For this review, take the finished solid that the model builds, in its own axes (mm). A direction names the side the tool comes from. Round coordinates to 2 decimals unless told otherwise and drop trailing zeros. Loops run counter-clockwise (first coordinate to the right, second up) from the corner with the lowest first, then second, coordinate; pieces in that order, holes last. Notation, with made-up numbers: (49, -31) -> (74, -31) arc R10 cw to (74, -27) -> close; hole circle Ø9 at (75.25, -29.75). An arc over 180 degrees is marked (long way). Use one line per item in the form item = value. Start each with the question number.
Autodesk Inventor part; units mm, degrees
sketch "Sketch1" plane through (0, 0, 0) normal (0, 0, 1) x (1, 0, 0)
  line L0 (0, 2.868) -> (2, 2.868)
  line L1 (2, 2.868) -> (2, -21.132)
  line L2 (2, -21.132) -> (0, -21.132)
  line L3 (0, -21.132) -> (0, 2.868)
  line L4 (4, -23.132) -> (4, 4.868)
  line L5 (4, 4.868) -> (0, 4.868)
  line L6 (0, -23.132) -> (4, -23.132)
  line L7 (0, 2.868) -> (0, 4.868)
  line L8 (0, -23.132) -> (0, -21.132)
  line L9 (-30, 5.364) -> (-30, -29.5729)
  line L10 (-60, 2.868) -> (-62, 2.868)
  line L11 (-62, 2.868) -> (-62, -21.132)
  line L12 (-62, -21.132) -> (-60, -21.132)
  line L13 (-60, -21.132) -> (-60, 2.868)
  line L14 (-64, -23.132) -> (-64, 4.868)
  line L15 (-64, 4.868) -> (-60, 4.868)
  line L16 (-60, -23.132) -> (-64, -23.132)
  line L17 (-60, 2.868) -> (-60, 4.868)
  line L18 (-60, -23.132) -> (-60, -21.132)
  point P0 (0, 0)
  point P1 (-60, 0)
  dimension "d0" = 2
  dimension "d1" = 24
  dimension "d2" = 2
  dimension "d3" = 32
extrude "Extrusion1" add sketch "Sketch1" along normal blind 94.2 contours L7 L5 L4 L6 L8 L2 L1 L0 | L10 L11 L12 L18 L16 L14 L15 L17
sketch "Sketch3" plane through (-64, 4.868, 0) normal (0, 1, 0) x (1, 0, 0)
  line L0 (4, 0) -> (0, 0)
  line L1 (0, 0) -> (0, -94.2)
  line L2 (4, -94.2) -> (0, -94.2)
  line L3 (4, 0) -> (4, -94.2)
  line L4 (68, 0) -> (64, 0)
  line L5 (64, 0) -> (64, -94.2)
  line L6 (68, -94.2) -> (64, -94.2)
  line L7 (68, 0) -> (68, -94.2)
  line L8 (0, 0) -> (68, 0)
  line L9 (68, 0) -> (68, -94.2)
  line L10 (68, -94.2) -> (0, -94.2)
  line L11 (0, -94.2) -> (0, 0)
extrude "Extrusion2" add sketch "Sketch3" along normal blind 3
sketch "Sketch4" plane through (0, 0, 0) normal (0, 0, -1) x (-1, 0, 0)
  line L0 (0, 2.868) -> (-2, 2.868)
  line L1 (0, 4.868) -> (0, 2.868)
  line L2 (0, 4.868) -> (60, 4.868)
  line L3 (60, 2.868) -> (60, 4.868)
  line L4 (62, 2.868) -> (60, 2.868)
  line L5 (62, -21.132) -> (62, 2.868)
  line L6 (60, -21.132) -> (62, -21.132)
  line L7 (60, -23.132) -> (60, -21.132)
  line L8 (64, -23.132) -> (60, -23.132)
  line L9 (64, -23.132) -> (64, 7.868)
  line L10 (-4, 7.868) -> (64, 7.868)
  line L11 (-4, -23.132) -> (-4, 7.868)
  line L12 (0, -23.132) -> (-4, -23.132)
  line L13 (0, -21.132) -> (0, -23.132)
  line L14 (-2, -21.132) -> (0, -21.132)
  line L15 (-2, 2.868) -> (-2, -21.132)
  line L16 (-4, 7.868) -> (64, 7.868)
  line L17 (64, 7.868) -> (64, -23.132)
  line L18 (64, -23.132) -> (-4, -23.132)
  line L19 (-4, -23.132) -> (-4, 7.868)
  line L20 (0, -23.132) -> (0, 4.868)
  line L21 (0, 4.868) -> (60, 4.868)
  line L22 (60, -23.132) -> (60, 4.868)
  line L23 (60, -23.132) -> (60, -21.132)
  point P0 (0, 0)
extrude "Extrusion3" add sketch "Sketch4" against normal blind 2 contours L20 L14 L15 L0 | L0 L15 L14 L13 L12 L11 L10 L9 L8 L7 L6 L5 L4 L3 L2 L1 | L4 L5 L6 L22
sketch "Sketch7" plane through (4, -23.132, 94.2) normal (1, 0, 0) x (0, 0, -1)
  line L0 (2, 24) -> (90.2, 24)
  line L1 (90.2, 24) -> (90.2, 4)
  line L2 (90.2, 4) -> (2, 4)
  line L3 (2, 4) -> (2, 24)
  line L4 (92.2, 26) -> (92.2, 2)
  line L5 (92.2, 26) -> (0, 26)
  line L6 (0, 0) -> (0, 31)
  line L7 (92.2, 2) -> (0, 2)
  point P0 (94.2, 23.132)
  dimension "d12" = 2
  dimension "d13" = 2
  dimension "d14" = 2
  dimension "d15" = 2
extrude "Extrusion4" cut sketch "Sketch7" against normal up to surface (68 mm away) contours L0 L1 L2 L3
sketch "Sketch9" plane through (-64, -23.132, 0) normal (-1, 0, 0) x (0, 0, 1)
  line L0 (4, 4) -> (4, 24)
  line L1 (4, 24) -> (92.2, 24)
  line L2 (92.2, 24) -> (92.2, 4)
  line L3 (92.2, 4) -> (4, 4)
  line L4 (0, 0) -> (94.2, 0)
  line L5 (94.2, 0) -> (94.2, 31)
  line L6 (0, 31) -> (94.2, 31)
  line L7 (0, 0) -> (0, 31)
  point P0 (0, 23.132)
ref_plane "Work Plane1" through (-64, 2.868, 4) normal (1, 0, 0) x (0, 1, 0)
sketch "Sketch10" plane through (-64, 7.868, 0) normal (0, 1, 0) x (1, 0, 0)
  line L0 (0, 0) -> (0, -94.2)
  line L1 (68, 0) -> (0, 0)
  line L2 (0, -94.2) -> (68, -94.2)
  line L3 (0, 0) -> (0, -94.2)
  line L4 (0, -32.1) -> (0, 0)
  line L5 (0, 0) -> (0, -94.2)
  line L6 (0, -94.2) -> (68, -94.2)
  line L7 (68, -94.2) -> (68, 0)
  line L8 (68, 0) -> (0, 0)
  point P0 (64, 0)
  dimension "d36" = 0
sketch "Sketch11" plane through (-64, 7.868, 0) normal (0, 1, 0) x (1, 0, 0)
  line L0 (68, 0) -> (68, -94.2)
  point P0 (64, 0)
properties part number "kontroller2"
Item 1: Take a section at B-B on z = 59.5. Give the boundary of the cut face in (x, y), plus the area to 3 significant figures.
Item 2: Draft analysis for pull direction X (two halves, no side actions). For faces 6 (the flat face through (1, -9, 2)), 7 (the flat face through (3, 0.868, 49)), 8 (the flat face through (0, -22, 40)), 9 (the flat face through (-64, 1.5, 43.4)), state which applies: +X half, -X half, draft (parallel to the pull), parting line (faces both ways), or undercut.
Item 3: Take a section at A-A on y = -5.5. Give the boundary of the cut face in (x, z), plus the area to 3 significant figures.
Item 4: Take a section at C-C on x = -5. Give the boundary of the cut face in (y, z), plus the area to 3 significant figures.
Item 5: Wall thickness on line 1 (Y direction, x = 1, z = 55); line 2 (X direction, y = 1.5, z = 10.5); line 3 (X direction, y = 3.5, z = 83.5): over which ranges is each line inside the solid? List them lowest first.
Item 6: Machinability: for faces 1 (the flat face through (-63, -19.132, 47)), 2 (the flat face through (-30.2, 5.1, 0)), 3 (the flat face through (-30.2, 5.1, 94.2)), 4 (the flat face through (-61, -21.132, 47)), 5 (the flat face through (-60, -22, 40)), which of the approach directions +Z, -Z, +X, -X, +Y, -Y give a long, thin tool a straight path to every point of the face, cutting with its end or side? Answer none if there is none.
Item 7: For P1, Ø1.5, axis at x = -34, z = 18.5, coming from the -Y side; P2, Ø12, axis at x = -50.5, y = -13.5, coming from the -Z side; P3, Ø1.6, axis at x = -60.5, y = -4, coming from the +Z side, all flat-tipped, find the tip position at first contact; note any pin that passes through.
Results:
q1.outline = (-64, -23.13) -> (-60, -23.13) -> (-60, -21.13) -> (-62, -21.13) -> (-62, -19.13) -> (-64, -19.13) -> close; (-64, 0.87) -> (-62, 0.87) -> (-62, 2.87) -> (-60, 2.87) -> (-60, 4.87) -> (0, 4.87) -> (0, 2.87) -> (2, 2.87) -> (2, 0.87) -> (4, 0.87) -> (4, 7.87) -> (-64, 7.87) -> close; (0, -23.13) -> (4, -23.13) -> (4, -19.13) -> (2, -19.13) -> (2, -21.13) -> (0, -21.13) -> close
q1.area = 252 mm2
q2.face_6 = undercut
q2.face_7 = draft
q2.face_8 = undercut
q2.face_9 = -X half
q3.outline = (-64, 0) -> (-60, 0) -> (-60, 2) -> (-62, 2) -> (-62, 4) -> (-64, 4) -> close; (-64, 92.2) -> (-62, 92.2) -> (-62, 94.2) -> (-64, 94.2) -> close; (0, 0) -> (4, 0) -> (4, 4) -> (2, 4) -> (2, 2) -> (0, 2) -> close; (2, 92.2) -> (4, 92.2) -> (4, 94.2) -> (2, 94.2) -> close
q3.area = 32.0 mm2
q4.outline = (4.87, 0) -> (7.87, 0) -> (7.87, 94.2) -> (4.87, 94.2) -> close
q4.area = 283 mm2
q5.line_1 = -23.13 to -21.13, 2.87 to 7.87
q5.line_2 = -64 to -62, 2 to 4
q5.line_3 = -64 to -60, 0 to 4
q6.face_1 = +X, -X
q6.face_2 = -Z, +X, -X, +Y, -Y
q6.face_3 = +Z, +X, -X, +Y, -Y
q6.face_4 = +Z
q6.face_5 = +Z, -Z, -Y
q7.P1 = 4.87
q7.P2 = through
q7.P3 = 2
